Source: CAD feature listing. Evaluate the final solid. Frame: model axes, mm. A direction names the side the tool comes from. Give positions to 0.01 mm unless a question says otherwise; leave off trailing zeros. Write each loop counter-clockwise with the first axis right and the second up, starting at its lowest first coordinate (ties: lowest second). Pieces come first, ordered by that corner, then holes.
```python
from build123d import *

# Parameters (mm, degrees)
SKETCH3_R               = 8
BOSS_EXTRUDE1_DEPTH     = 20
SKETCH4_R               = 4
CUT_EXTRUDE1_DEPTH      = 12
CUT_EXTRUDE2_DEPTH      = 23.978250586
CUT_EXTRUDE2_DEPTH_BACK = 23.978250586
SKETCH5_R               = 1.5


with BuildPart() as part:
    # Sketch3 → Boss-Extrude1 (new body)
    with BuildSketch(Plane(origin=(0, 0, 0), x_dir=(1, 0, 0), z_dir=(0, 1, 0))):
        with Locations(Location((0, 0, 0), (0, 0, 270))):
            Circle(SKETCH3_R)
    extrude(amount=BOSS_EXTRUDE1_DEPTH)

    # Sketch4 → Cut-Extrude1 (cut)
    with BuildSketch(Plane.XZ):
        with Locations(Location((0, 0, 0), (0, 0, 270))):
            Circle(SKETCH4_R)
    extrude(amount=-CUT_EXTRUDE1_DEPTH, mode=Mode.SUBTRACT)

    # Sketch5 → Cut-Extrude2 (cut, two sides: drawn at the far end of the back side and taken through both)
    with BuildSketch(Plane(origin=(0, 0, 0), x_dir=(0, 0, -1), z_dir=(1, 0, 0)).offset(-CUT_EXTRUDE2_DEPTH_BACK)):
        with Locations((0, 2.5)):
            Circle(SKETCH5_R)
    extrude(amount=CUT_EXTRUDE2_DEPTH + CUT_EXTRUDE2_DEPTH_BACK, mode=Mode.SUBTRACT)


solid = part.part
```
1. Line query: probe 1 along X at (y, z) = (6.75, 0); probe 2 along Y at (x, z) = (5.7, 0); probe 3 along Z at (x, y) = (0.25, 7). Output: solid intervals per line, ascending.
2. Section query C-C (x = -6.5). Return loops of the section in (y, z), plus the area to 3 significant figures.
3. Section query B-B (x = 0). Return loops of the section in (y, z), plus the area to 3 significant figures.
4. Pull-direction query (Z, two-part tool) for faces 3 (the cylindrical face through (-1.532, 5.916, -3.695)), 4 (the cylindrical face through (-5.886, 1.925, -1.386)), 5 (the flat face through (-2, 0, -4)), 6 (the cylindrical face through (-7.81, 9.86, -1.73)); classes: pulls with the +Z half, pulls with the -Z half, needs draft (parallel to the pull), parting line crosses it, or undercut.
5. Pin query (flat end, axial travel): P1, Ø1.5, axis at y = 10, z = -3, coming from the +X side; P2, Ø1.5, axis at y = 15.5, z = -2, coming from the +X side; P3, Ø1.5, axis at y = 16.5, z = -2, coming from the -X side; P4, Ø2.5, axis at y = 2.5, z = 0, coming from the +X side. Return the tip coordinate at first contact, or that it passes through.
6. Access query for faces 1 (the flat face through (0, 20, 0)), 2 (the flat face through (0, 12, 0)). Directions: +Z, -Z, +X, -X, +Y, -Y. A direction counts if a zero-diameter tool reaches every point of the face in a straight line with its end or side. Return the directions, or none.
7. Section query A-A (z = 0). Return loops of the section in (x, y), plus the area to 3 significant figures.
8. Section query D-D (y = 15). Return loops of the section in (x, z).
The answers:
1. probe 1: x = -8 to -4, 4 to 8
1. probe 2: y = 0 to 1, 4 to 20
1. probe 3: z = -8 to -3.99, 3.99 to 8
2. outline: (0, -4.66) - (20, -4.66) - (20, 4.66) - (0, 4.66) - close; hole circle Ø3 at (2.5, 0)
2. area: 179 mm2
3. outline: (0, -8) - (20, -8) - (20, 8) - (0, 8) - (0, 4) - (12, 4) - (12, -4) - (0, -4) - close
3. area: 224 mm2
4. face 3: undercut
4. face 4: undercut
4. face 5: needs draft
4. face 6: parting line crosses it
5. P1: stops at x = 7.68
5. P2: stops at x = 7.9
5. P3: stops at x = -7.9
5. P4: passes through
6. face 1: +Z, -Z, +X, -X, +Y
6. face 2: -Y
7. outline: (-8, 0) - (-4, 0) - (-4, 1) - (-8, 1) - close; (-8, 4) - (-4, 4) - (-4, 12) - (4, 12) - (4, 4) - (8, 4) - (8, 20) - (-8, 20) - close; (4, 0) - (8, 0) - (8, 1) - (4, 1) - close
7. area: 200 mm2
8. outline: circle Ø16 at (0, 0)
